Could you check a few things on this model? Use its own coordinates, in mm. Face numbers are marked on the shaded views. A direction names the side the tool comes from. Give positions to 0.01 mm unless a question says otherwise; leave off trailing zeros. Write each loop counter-clockwise with the first axis right and the second up, starting at its lowest first coordinate (ties: lowest second). Pieces come first, ordered by that corner, then holes. Notation, with made-up numbers: (-10, 15) - (9, 15) arc R17 ccw to (9, 19) - close; hole circle Ø5 at (51, -16.75). An arc over 180 degrees is marked (long way). Answer in a Markdown table with one row per item.
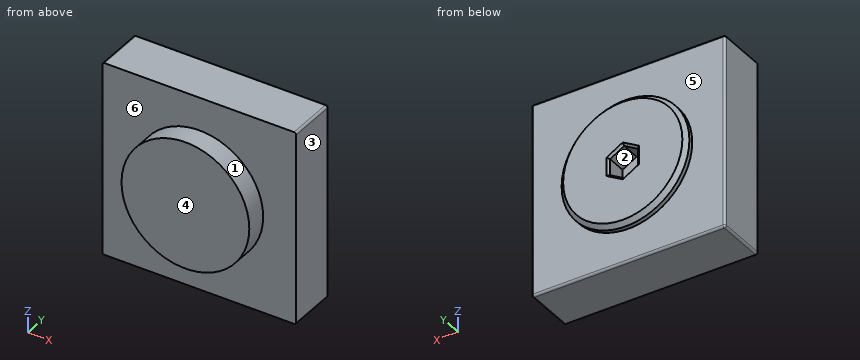
from build123d import *

# Parameters (mm, degrees)
SKETCH1_W           = 45.5
SKETCH1_H           = 45.5
BOSS_EXTRUDE1_DEPTH = 11.7
SKETCH2_R           = 15
BOSS_EXTRUDE2_DEPTH = 2
CHAMFER1_SIZE       = 1
CUT_EXTRUDE1_DEPTH  = 5
CHAMFER2_SIZE       = 0.5
FILLET1_R           = 0.5
SKETCH4_R           = 15
BOSS_EXTRUDE3_DEPTH = 5


with BuildPart() as part:
    # Sketch1 → Boss-Extrude1 (new body)
    with BuildSketch(Plane(origin=(0, 0, 0), x_dir=(1, 0, 0), z_dir=(0, 1, 0))):
        Rectangle(SKETCH1_W, SKETCH1_H)
    extrude(amount=BOSS_EXTRUDE1_DEPTH)

    # Sketch2 → Boss-Extrude2 (add)
    with BuildSketch(Plane(origin=(0, 11.7, 0), x_dir=(1, 0, 0), z_dir=(0, 1, 0))):
        Circle(SKETCH2_R)
    extrude(amount=BOSS_EXTRUDE2_DEPTH)

    # Chamfer1
    chamfer1_edges = [part.edges().sort_by_distance(p)[0] for p in [
        (-15, 13.7, 0),
    ]]
    chamfer(chamfer1_edges, length=CHAMFER1_SIZE)

    # Sketch3 → Cut-Extrude1 (cut)
    with BuildSketch(Plane(origin=(0, 13.7, 0), x_dir=(1, 0, 0), z_dir=(0, 1, 0))):
        Polygon((0, 3.810511777), (-3.3, 1.905255888), (-3.3, -1.905255888), (0, -3.810511777), (3.3, -1.905255888), (3.3, 1.905255888), align=None)
    extrude(amount=-CUT_EXTRUDE1_DEPTH, mode=Mode.SUBTRACT)

    # Chamfer2
    chamfer2_edges = [part.edges().sort_by_distance(p)[0] for p in [
        (1.65, 13.7, -2.857883832),
        (-1.65, 13.7, -2.857883832),
        (-3.3, 13.7, 0),
        (-1.65, 13.7, 2.857883832),
        (1.65, 13.7, 2.857883832),
        (3.3, 13.7, 0),
    ]]
    chamfer(chamfer2_edges, length=CHAMFER2_SIZE)

    # Fillet1
    fillet1_edges = [part.edges().sort_by_distance(p)[0] for p in [
        (-22.75, 11.7, 0),
        (0, 11.7, 22.75),
        (22.75, 11.7, 0),
        (22.75, 5.85, 22.75),
        (-22.75, 5.85, 22.75),
        (-22.75, 5.85, -22.75),
        (22.75, 5.85, -22.75),
        (0, 11.7, -22.75),
    ]]
    fillet(fillet1_edges, radius=FILLET1_R)

    # Sketch4 → Boss-Extrude3 (add)
    with BuildSketch(Plane(origin=(0, 0, 0), x_dir=(-1, 0, 0), z_dir=(0, -1, 0))):
        Circle(SKETCH4_R)
    extrude(amount=BOSS_EXTRUDE3_DEPTH)


solid = part.part
1) Imagine slicing it at A-A (y = 10). List the corners of the cut face in (x, z) for me.
Check values:
| item | result |
|---|---|
| outline | (-22.75, -22.25) arc R0.5 ccw to (-22.25, -22.75) - (22.25, -22.75) arc R0.5 ccw to (22.75, -22.25) - (22.75, 22.25) arc R0.5 ccw to (22.25, 22.75) - (-22.25, 22.75) arc R0.5 ccw to (-22.75, 22.25) - close; hole (-3.3, -1.91) - (0, -3.81) - (3.3, -1.91) - (3.3, 1.91) - (0, 3.81) - (-3.3, 1.91) - close |
2) If I drill on line 1 (Y direction, x = -19, z = -19.5); line 2 (X direction, y = -0.25, z = -1.5), over which ranges is the centre line in solid material (lowest first)?
Check values:
| item | result |
|---|---|
| line 1 | y = 0 to 11.7 |
| line 2 | x = -14.92 to 14.92 |
3) Will these pins go through, and if not, where does the flat tip stop? P1, Ø4, axis at x = -16, z = -12.5, coming from the -Y side; P2, Ø2, axis at x = 0, z = 0.5, coming from the +Y side; P3, Ø2, axis at x = -14, y = -2.5, coming from the +Z side.
Check values:
| item | result |
|---|---|
| P1 | stops at y = 0 |
| P2 | stops at y = 8.7 |
| P3 | stops at z = 7.48 |
4) On a 3-axis mill with a long thin cutter (end or side, diameter ignored), from which of +Z, -Z, +X, -X, +Y, -Y can I reach the whole of each face in a straight line? I mean the marked faces 4, 5 and 6. Say none if no direction works.
Check values:
| item | result |
|---|---|
| face 4 | +Z, -Z, +X, -X, -Y |
| face 5 | +Y |
| face 6 | -Y |
5) Imagine slicing it at B-B (z = 0). List the corners of the cut face in (x, y) for me.
Check values:
| item | result |
|---|---|
| outline | (-22.75, 0) - (-15, 0) - (-15, -5) - (15, -5) - (15, 0) - (22.75, 0) - (22.75, 11.2) arc R0.5 ccw to (22.25, 11.7) - (15, 11.7) - (15, 12.7) - (14, 13.7) - (3.8, 13.7) - (3.3, 13.2) - (3.3, 8.7) - (-3.3, 8.7) - (-3.3, 13.2) - (-3.8, 13.7) - (-14, 13.7) - (-15, 12.7) - (-15, 11.7) - (-22.25, 11.7) arc R0.5 ccw to (-22.75, 11.2) - close |
6) Imagine slicing it at C-C (x = -17.5). List the corners of the cut face in (y, z) for me, then the cut area to 3 significant figures.
Check values:
| item | result |
|---|---|
| outline | (0, -22.75) - (11.2, -22.75) arc R0.5 ccw to (11.7, -22.25) - (11.7, 22.25) arc R0.5 ccw to (11.2, 22.75) - (0, 22.75) - close |
| area | 532 mm2 |
7) We'd pull the mould along X, two halves only. Please class the marked faces 1, 2 and 3: +X half, -X half, draft (parallel to the pull), parting line (faces both ways), or undercut.
Check values:
| item | result |
|---|---|
| face 1 | parting line |
| face 2 | undercut |
| face 3 | +X half |
